The model under review builds one solid part; all positions refer to its coordinate system, in mm. A direction names the side the tool comes from. Coordinates: 2 decimals unless noted, no trailing zeros. Write each loop counter-clockwise with the first axis right and the second up, starting at its lowest first coordinate (ties: lowest second). Pieces come first, ordered by that corner, then holes. Notation, with made-up numbers: (1, -21.75) - (34, -21.75) arc R26 ccw to (34, -0.75) - close; hole circle Ø4 at (6.25, 42.5). An arc over 180 degrees is marked (long way). Return JSON: item names as keys, results as strings. Group by question number.
(1) For pin 1 Ø4 at (x, z) = (4.5, -18.5) entering from -Y; pin 2 Ø4 at (x, z) = (-1.5, -48.5) entering from -Y; pin 3 Ø1 at (x, y) = (4, 7) entering from -Z, all flat-tipped, find the tip position at first contact; note any pin that passes through.
(2) We need section C-C on x = -1.5. State the section outline as (y, z) points.
(3) Draft analysis for pull direction Y (two halves, no side actions). For faces 3 (the face through (3, -27.5, 18)), 4 (the face through (3.04, -12.57, 22.35)), 5 (the face through (3, 0, -60)), state which applies: released by +Y, released by -Y, zero draft, split by the parting line, or undercut.
(4) Tool access review of faces 1 (the face through (-3.45, 6.07, -29.51)), 2 (the face through (2.958, 21.595, -23.606)): name each direction out of +Z, -Z, +X, -X, +Y, -Y from which nothing blocks a thin tool from reaching the whole face with its end or side.
(5) To check wall thickness, follow L1, parallel to Y at x = 3.85, z = 23; L2, parallel to X at y = -13, z = -10; L3, parallel to Z at x = 4.5, y = -2. State the ranges of each line that lie inside material, in increasing order. Write a range as from..to.
(6) We need section B-B on z = -32. State the section outline as (x, y) points, then the cut area to 3 significant figures.
(7) We need section D-D on z = 12.5. State the section outline as (x, y) points, then the cut area to 3 significant figures.
Autodesk Inventor part; units mm, degrees
ref_plane "YZ Plane" through (0, 0, 0) normal (1, 0, 0) x (0, 1, 0)
ref_plane "XZ Plane" through (0, 0, 0) normal (0, 1, 0) x (-1, 0, 0)
ref_plane "XY Plane" through (0, 0, 0) normal (0, 0, 1) x (1, 0, 0)
sketch "Sketch1" plane through (0, 0, 0) normal (1, 0, 0) x (0, 1, 0)
  line L0 (27.5, 35) -> (-27.5, 35)
  line L1 (-27.5, 35) -> (-27.5, 0)
  line L2 (-27.5, 0) -> (-15.5217, -47.8829)
  arc A0 (-15.5217, -47.8829) -> (15.5217, -47.8829) centre (0, -44) ccw
  line L3 (27.5, 35) -> (27.5, 0)
  line L4 (27.5, 0) -> (15.5217, -47.8829)
  line L5 (-38.5, 0) -> (38.5, 0) construction
  line L6 (0, -79) -> (0, 54) construction
  circle A1 centre (0, -44) radius 9
  point P0 (0, 0)
  point P1 (0, -60)
  dimension "d0" = 55
  dimension "d1" = 35
  dimension "d2" = 18
  dimension "d3" = 16
  dimension "d4" = 60
extrude "Extrusion1" add sketch "Sketch1" along normal blind 6 contours L3 L4 A0 L2 L1 L0 | A1
sketch "Sketch2" plane through (0, 0, 0) normal (-1, 0, 0) x (0, 0, 1)
  circle A0 centre (-44.1499, 0) radius 15.8501
  arc A1 (-47.8829, 15.5217) -> (-47.8829, -15.5217) centre (-44, 0) ccw construction
  point P0 (0, 0)
extrude "Extrusion2" add sketch "Sketch2" along normal blind 7
hole "Hole1" at (0, 15.5, 23) direction (1, 0, 0) diameter 6 end through all
hole "Hole2" at (0, -15.5, 23) direction (1, 0, 0) diameter 6 end through all
properties part number "collar"
Ans:
{
 "1": {"pin 1": "y = -23.37", "pin 2": "y = -15.7", "pin 3": "z = -58.62"},
 "2": {"outline": "circle Ø31.7 at (0, -44.15)"},
 "3": {"face 3": "released by -Y", "face 4": "undercut", "face 5": "split by the parting line"},
 "4": {"face 1": "-X", "face 2": "-Z, +X, -X, +Y"},
 "5": {"L1": "-27.5..-18.5, -12.5..12.5, 18.5..27.5", "L2": "0..6", "L3": "-59.87..35"},
 "6": {"outline": "(-7, -10.18) - (0, -10.18) - (0, -19.49) - (6, -19.49) - (6, 19.49) - (0, 19.49) - (0, 10.18) - (-7, 10.18) - close", "area": "376 mm²"},
 "7": {"outline": "(0, -27.5) - (6, -27.5) - (6, 27.5) - (0, 27.5) - close", "area": "330 mm²"}
}
